The model under review builds one solid part; all positions refer to its coordinate system, in mm. Round coordinates to 2 decimals unless told otherwise and drop trailing zeros. Write each loop counter-clockwise with the first axis right and the second up, starting at its lowest first coordinate (ties: lowest second). Pieces come first, ordered by that corner, then holes. Notation, with made-up numbers: M 70.25,-40 L 121.25,-40 A19 ccw 121.25,-29 Z; hole C 15,42 d4. An arc over 180 degrees is marked long. Write item = value, one per line. Start each with the question number.
Item 1: To check wall thickness, follow line 1 along Z through (x, y) = (168, -30); line 2 along X through (y, z) = (-35.5, 4); line 3 along X through (y, z) = (-25.5, 2.5). State the ranges of each line that lie inside material, in increasing order.
Item 2: For pin 1 Ø10 at (y, z) = (-29.8, 29.8) entering from -X; pin 2 Ø12 at (x, y) = (585, -14.5) entering from +Z; pin 3 Ø4 at (y, z) = (-21.5, 23) entering from -X; pin 4 Ø8 at (x, z) = (331, 7.5) entering from -Y, all flat-tipped, find the tip position at first contact; note any pin that passes through.
Item 3: The part is to be moulded in two halves that separate along Y. For faces 1 (the cylindrical face through (374.154, -16.904, 39.496)), 2 (the cylindrical face through (375.709, -31.648, 21.495)), 3 (the flat face through (762, -29, 17)), say which applies: +Y half, -Y half, draft (parallel to the pull), parting line (faces both ways), or undercut.
Item 4: Take a section at A-A, the plane x = 551. Give the boundary of the cut face in (y, z), plus the area to 3 significant figures.
from build123d import *

# Parameters (mm, degrees)
F0_R     = 21.4571011733
F0_R_2   = 8.5102706454
F1_DEPTH = 762


# Not quite as in the source:
# - a fillet or chamfer that OpenCascade refuses, or shapes differently, is made with other operations: its cross-section is extruded or revolved along the edge and cut away or added


with BuildPart() as f1:
    # F0 (on Right) → F1 (new body)
    with BuildSketch(Plane.YZ):
        with Locations((-28.4389311976, 21.4029382453)):
            Circle(F0_R)
        with Locations((-29.8031512648, 29.8031531274)):
            Circle(F0_R_2, mode=Mode.SUBTRACT)
    extrude(amount=F1_DEPTH)

    # F2: fillet of radius 3.0660512242 on 4 edges, made by hand


with BuildPart() as f2_tool1:
    # F2_s2 → F2_t3 (revolve)
    with BuildSketch(Plane.XY.offset(21.4029382453)):
        with BuildLine():
            ThreePointArc((758.9339487758, -6.9818300243), (761.1019743879, -7.8798556364), (762, -10.0478812485))
            Line((762, -10.0478812485), (762, -6.9818300243))
            Line((762, -6.9818300243), (758.9339487758, -6.9818300243))
        make_face()
    revolve(axis=Axis((762, -28.4389311976, 21.4029382453), (1, 0, 0)))


with BuildPart() as f2_tool4:
    # F2_s5 → F2_t6 (revolve)
    with BuildSketch(Plane.XY.offset(29.8031531274)):
        with BuildLine():
            ThreePointArc((758.9339487758, -21.2928806194), (761.1019743879, -20.3948550073), (762, -18.2268293951))
            Line((762, -18.2268293951), (762, -21.2928806194))
            Line((762, -21.2928806194), (758.9339487758, -21.2928806194))
        make_face()
    revolve(axis=Axis((762, -29.8031512648, 29.8031531274), (1, 0, 0)))


with BuildPart() as f2_tool7:
    # F2_s8 → F2_t9 (revolve)
    with BuildSketch(Plane.XY.offset(29.8031531274)):
        with BuildLine():
            ThreePointArc((3.0660512242, -21.2928806194), (0.8980256121, -20.3948550073), (0, -18.2268293951))
            Line((0, -18.2268293951), (0, -21.2928806194))
            Line((0, -21.2928806194), (3.0660512242, -21.2928806194))
        make_face()
    revolve(axis=Axis((0, -29.8031512648, 29.8031531274), (1, 0, 0)))


with BuildPart() as f1_1:
    add(f1.part)

    # F2_t10: cut F2_tool1, F2_tool4, F2_tool7
    add([f2_tool1.part, f2_tool4.part, f2_tool7.part], mode=Mode.SUBTRACT)


solid = f1_1.part
Response values:
q1.line_1 = 0 to 21.3, 38.31 to 42.8
q1.line_2 = 0 to 761.98
q1.line_3 = 0 to 761.91
q2.pin_1 = through
q2.pin_2 = 41.34
q2.pin_3 = 0
q2.pin_4 = -47.47
q3.face_1 = parting line
q3.face_2 = undercut
q3.face_3 = draft
q4.outline = C -28.44,21.4 d42.91; hole C -29.8,29.8 d17.02
q4.area = 1,220 mm2
